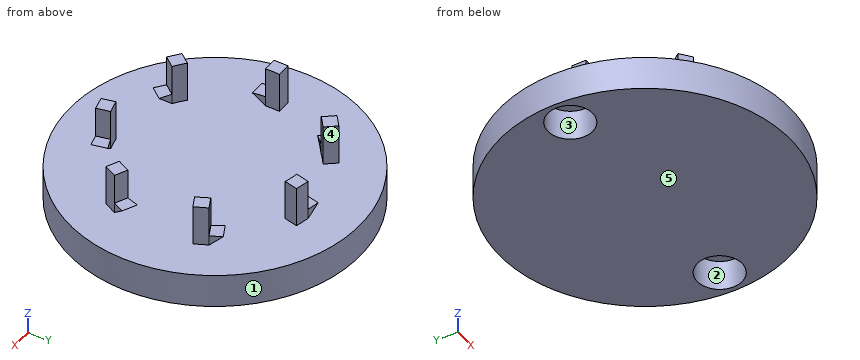
from build123d import *

# Parameters (mm, degrees)
F0_R            = 21.5
F0_R_2          = 13.5
F1_DEPTH        = 5
F3_DEPTH        = 6
F4_R            = 3.325
F5_DEPTH        = 4.5
F7_END_RADIUS   = 13.5
F7_REACH        = 39.2960714607
F7_COPIES_COUNT = 7


# Not quite as in the source:
# - a pattern or mirror of a feature is missing from the dataset's text; its kind, count and spacing are read off the source's solid


with BuildPart() as f1:
    # F0 (on Top) → F1 (new body)
    with BuildSketch(Plane.XY):
        Circle(F0_R)
        Circle(F0_R_2, mode=Mode.SUBTRACT)
        Circle(F0_R_2)
    extrude(amount=F1_DEPTH)

    # F2 (on face) → F3 (join)
    with BuildSketch(Plane.XY.offset(5)):
        with BuildLine():
            ThreePointArc((-13.4614857204, -1.0190202158), (-13.5, 0), (-13.4614857204, 1.0190202158))
            Line((-13.4614857204, 1.0190202158), (-15.4614857204, 1.0190202158))
            Line((-15.4614857204, 1.0190202158), (-15.4614857204, -1.0190202158))
            Line((-15.4614857204, -1.0190202158), (-13.4614857204, -1.0190202158))
        make_face()
        with BuildLine():
            ThreePointArc((-7.5963969786, -11.1599620494), (-8.4171123251, -10.5547250133), (-9.1898011505, -9.8892646246))
            Line((-9.1898011505, -9.8892646246), (-10.4367807542, -11.4529275895))
            Line((-10.4367807542, -11.4529275895), (-8.8433765823, -12.7236250143))
            Line((-8.8433765823, -12.7236250143), (-7.5963969786, -11.1599620494))
        make_face()
        with BuildLine():
            ThreePointArc((3.9889336264, -12.8972248381), (3.0040326084, -13.1615268145), (2.0019911235, -13.3507314984))
            Line((2.0019911235, -13.3507314984), (2.4470329914, -15.3005873227))
            Line((2.4470329914, -15.3005873227), (4.4339754943, -14.8470806625))
            Line((4.4339754943, -14.8470806625), (3.9889336264, -12.8972248381))
        make_face()
        with BuildLine():
            ThreePointArc((12.5705158512, -4.9226142683), (12.1630797167, -5.8574304781), (11.6862432483, -6.7588252486))
            Line((11.6862432483, -6.7588252486), (13.4881809841, -7.6265927268))
            Line((13.4881809841, -7.6265927268), (14.372453587, -5.7903817465))
            Line((14.372453587, -5.7903817465), (12.5705158512, -4.9226142683))
        make_face()
        with BuildLine():
            ThreePointArc((11.6862432483, 6.7588252486), (12.1630797167, 5.8574304781), (12.5705158512, 4.9226142683))
            Line((12.5705158512, 4.9226142683), (14.372453587, 5.7903817465))
            Line((14.372453587, 5.7903817465), (13.4881809841, 7.6265927268))
            Line((13.4881809841, 7.6265927268), (11.6862432483, 6.7588252486))
        make_face()
        with BuildLine():
            ThreePointArc((2.0019911235, 13.3507314984), (3.0040326084, 13.1615268145), (3.9889336264, 12.8972248381))
            Line((3.9889336264, 12.8972248381), (4.4339754943, 14.8470806625))
            Line((4.4339754943, 14.8470806625), (2.4470329914, 15.3005873227))
            Line((2.4470329914, 15.3005873227), (2.0019911235, 13.3507314984))
        make_face()
        with BuildLine():
            ThreePointArc((-9.1898011505, 9.8892646246), (-8.4171123251, 10.5547250133), (-7.5963969786, 11.1599620494))
            Line((-7.5963969786, 11.1599620494), (-8.8433765823, 12.7236250143))
            Line((-8.8433765823, 12.7236250143), (-10.4367807542, 11.4529275895))
            Line((-10.4367807542, 11.4529275895), (-9.1898011505, 9.8892646246))
        make_face()
    extrude(amount=F3_DEPTH)

    # F4 (on face) → F5 (cut)
    with BuildSketch(Plane(origin=(0, 0, 0), x_dir=(1, 0, 0), z_dir=(0, 0, -1))):
        with Locations((-17.5, 0)):
            Circle(F4_R)
        with Locations((17.5, 0)):
            Circle(F4_R)
    extrude(amount=-F5_DEPTH, mode=Mode.SUBTRACT)

    f7_end = (Plane(origin=(0, 0, 8), x_dir=(-1, 0, 0), z_dir=(0, 0, -1)) * Cylinder(F7_END_RADIUS, 202.1882593652, mode=Mode.PRIVATE)).faces().sort_by_distance((-13.5, 0, 8))[0]
    # F6 (on face) → F7 (join, up to the whole of a round face its end follows)
    with BuildSketch(Plane(origin=(-15.4614857204, 0, 0), x_dir=(0, -1, 0), z_dir=(-1, 0, 0))):
        Polygon((1.0190202158, 6.5), (1.0190202158, 5), (2.8066506047, 6.5), align=None)
    f7_long = extrude(amount=-F7_REACH, mode=Mode.PRIVATE)
    f7 = split(f7_long, bisect_by=f7_end, keep=Keep.ALL, mode=Mode.PRIVATE).solids().sort_by_distance((-15.4614857204, -1.6148970121, 6))[0]
    add(f7)

    # F7_copies: F7 ×7 about axis
    f7_copies_axis = Axis((0, 0, 0), (0, 0, 1))
    for i in range(1, F7_COPIES_COUNT):
        add(f7.rotate(f7_copies_axis, i * 360 / F7_COPIES_COUNT))


solid = f1.part
Build history of the part. All positions in model axes, mm. Face numbers are marked on the shaded views. A direction names the side the tool comes from. Coordinates: 2 decimals unless noted, no trailing zeros. Order: outer loops, then holes, each group sorted by start corner. A loop starts at its lowest first (then second) coordinate and runs counter-clockwise, first axis right, second up. Notation, with made-up numbers: (40, 60.5) - (94, 60.5) arc R15 cw to (94, 75.5) - close; hole circle Ø8 at (-10.5, 36.25). An arc over 180 degrees is marked (long way). Put each result on its own line as item: value.
1. Saw through at A-A (z = 10.25). Write the cut outline in (x, y).
Answer sheet:
outline: (-15.46, -1.02) - (-13.46, -1.02) arc R13.5 cw to (-13.46, 1.02) - (-15.46, 1.02) - close; (-10.44, -11.45) - (-8.84, -12.72) - (-7.6, -11.16) arc R13.5 cw to (-9.19, -9.89) - close; (-10.44, 11.45) - (-9.19, 9.89) arc R13.5 cw to (-7.6, 11.16) - (-8.84, 12.72) - close; (2, -13.35) - (2.45, -15.3) - (4.43, -14.85) - (3.99, -12.9) arc R13.5 cw to start; (2, 13.35) arc R13.5 cw to (3.99, 12.9) - (4.43, 14.85) - (2.45, 15.3) - close; (11.69, -6.76) - (13.49, -7.63) - (14.37, -5.79) - (12.57, -4.92) arc R13.5 cw to start; (11.69, 6.76) arc R13.5 cw to (12.57, 4.92) - (14.37, 5.79) - (13.49, 7.63) - close
2. Saw through at C-C (x = -17.5). Write the cut outline in (y, z) (3 decimals).
Answer sheet:
outline: (-12.49, 0) - (-3.325, 0) - (-3.325, 4.5) - (3.325, 4.5) - (3.325, 0) - (12.49, 0) - (12.49, 5) - (-12.49, 5) - close
3. Drop flat-ended pins along their axis: P1, Ø6, axis at y = 3.5, z = 2, coming from the -X side; P2, Ø7.5, axis at x = -17.5, y = -1, coming from the -Z side; P3, Ø0.7, axis at x = 12, y = 8, coming from the +Z side; P4, Ø1.6, axis at x = -15, z = 8, coming from the -Y side. Give the stop position or say it passes through.
Answer sheet:
P1: stops at x = -21.49
P2: stops at z = 0
P3: stops at z = 6.5
P4: stops at y = -1.02
4. Pull direction X, two halves, no side cores. Call the marked faces 3, 4 and 5: pulls with the +X half, pulls with the -X half, needs draft (parallel to the pull), parting line crosses it, or undercut.
Answer sheet:
face 3: undercut
face 4: pulls with the +X half
face 5: needs draft
5. Saw through at B-B (y = 0). Write the cut outline in (x, z) (3 decimals).
Answer sheet:
outline: (-21.5, 0) - (-20.825, 0) - (-20.825, 4.5) - (-14.175, 4.5) - (-14.175, 0) - (14.175, 0) - (14.175, 4.5) - (20.825, 4.5) - (20.825, 0) - (21.5, 0) - (21.5, 5) - (-13.5, 5) - (-13.5, 11) - (-15.461, 11) - (-15.461, 5) - (-21.5, 5) - close
6. Saw through at D-D (z = 3). Write the cut outline in (x, y) (3 decimals), and give its area (3 significant figures).
Answer sheet:
outline: circle Ø43 at (0, 0); hole circle Ø6.65 at (-17.5, 0); hole circle Ø6.65 at (17.5, 0)
area: 1,380 mm^2
7. Probe line 1 along Z through (x, y) = (-12, -16); line 2 along Y through (x, z) = (-8.5, 5.5); line 3 along Y through (x, z) = (17.5, 1.8) (3 decimals). List the from-to ranges inside material, lowest first. Write a range as [from, to].
Answer sheet:
line 1: z = [0, 5]
line 2: y = [-13, -10.49], [10.49, 12.29]
line 3: y = [-12.49, -3.325], [3.325, 12.49]
8. Tool access for the marked faces 1 and 2: list every direction of +Z, -Z, +X, -X, +Y, -Y with a clear straight run to the whole face (end or side of a thin tool).
Answer sheet:
face 1: +Z, -Z
face 2: -Z
